Verification items for this drawing (mm, ordinates from the low corner). A direction names the side the tool comes from. Coordinates: 2 decimals unless noted, no trailing zeros. Order: outer loops, then holes, each group sorted by start corner. A loop starts at its lowest first (then second) coordinate and runs counter-clockwise, first axis right, second up. Notation, with made-up numbers: M -39,68 L -12,68 A9 ccw -12,72 Z; hole C 13,39.25 d6. An arc over 180 degrees is marked long. Return JSON: item names as keys, results as strings. Group by question number.
1. Gauge pin test, flat ends, axial feed: pin 1 (5.5 mm diameter, centred on x = 13.5, z = 12, fed in from -Y); pin 2 (12 mm diameter, centred on y = 17.5, z = 17, fed in from +X). Record the tip position at first contact, or that the pin passes through.
2. Section check C-C, the plane z = 3. Record the cut outline in (x, y).
3. Section check B-B, the plane x = 16. Record the cut outline in (y, z), plus the area to 3 significant figures.
4. Section check D-D, the plane y = 19.5. Record the cut outline in (x, z).
5. Mould release check, pull along X, two halves, no side actions. Record for the marked faces 4, 5 and 6: +X half, -X half, draft (parallel to the pull), parting line (faces both ways), or undercut.
6. Set-up check for the marked faces 1, 2 and 3: record each of +Z, -Z, +X, -X, +Y, -Y from which the full face is reachable in a straight line by a thin tool's end or side.
7. Material ranges on line 1 along Z through (x, y) = (17, 10); line 2 along Y through (x, z) = (4.25, 16.5); line 3 along Z through (x, y) = (5.75, 28.5) (1 decimal), recorded low to high.
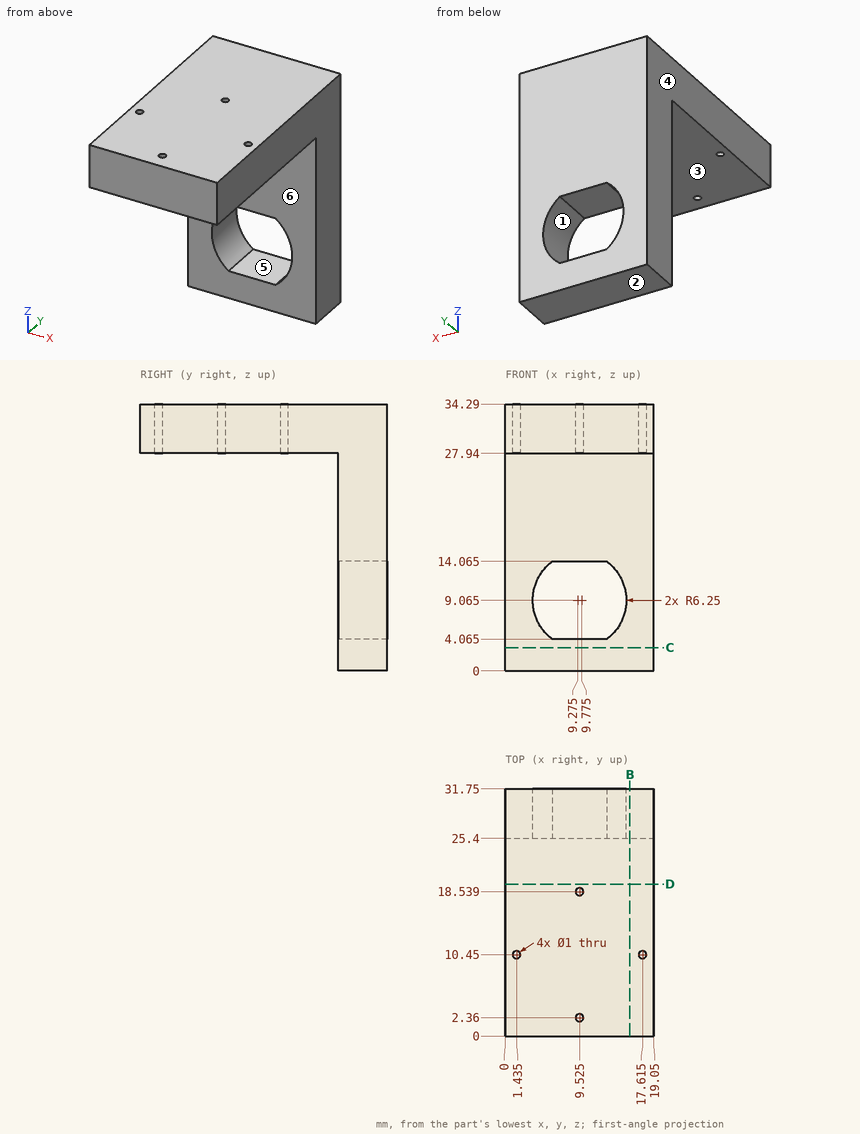
Answers follow:
{
 "1": {"pin 1": "y = 25.4", "pin 2": "through"},
 "2": {"outline": "M 0,25.4 L 19.05,25.4 L 19.05,31.75 L 0,31.75 Z"},
 "3": {"outline": "M 0,27.94 L 25.4,27.94 L 25.4,0 L 31.75,0 L 31.75,34.29 L 0,34.29 Z", "area": "379 mm^2"},
 "4": {"outline": "M 0,27.94 L 19.05,27.94 L 19.05,34.29 L 0,34.29 Z"},
 "5": {"face 4": "-X half", "face 5": "undercut", "face 6": "draft"},
 "6": {"face 1": "+Y, -Y", "face 2": "-Z, +X, -X, +Y, -Y", "face 3": "-Z, +X, -X, -Y"},
 "7": {"line 1": "27.94 to 34.29", "line 2": "25.4 to 31.75", "line 3": "0 to 4.3, 13.8 to 34.3"}
}
